The model under review builds one solid part; all positions refer to its coordinate system, in mm. Face numbers are marked on the shaded views. Give positions to 0.01 mm unless a question says otherwise; leave off trailing zeros. Loops run counter-clockwise (first coordinate to the right, second up) from the corner with the lowest first, then second, coordinate; pieces in that order, holes last. Notation, with made-up numbers: M 41,37.25 L 74,37.25 A20 cw 74,56.25 Z; hole C 60.5,-32 d5. An arc over 180 degrees is marked long. Put each result on its own line as item: value. Start each with the question number.
```python
from build123d import *

# Parameters (mm, degrees)
SKETCH1_R                               = 195
SKETCH1_R_2                             = 77.5
BOSS_EXTRUDE1_DEPTH                     = 5
SKETCH1_R_3                             = 67.5
SKETCH1_R_4                             = 25
BOSS_EXTRUDE1_2_DEPTH                   = 5
SKETCH1_4_R                             = 200
SKETCH1_4_R_2                           = 195
BOSS_EXTRUDE2_DEPTH                     = 147
SKETCH1_5_R                             = 77.5
SKETCH1_5_R_2                           = 67.5
BOSS_EXTRUDE3_DEPTH                     = 147
SKETCH1_6_R                             = 25
BOSS_EXTRUDE4_DEPTH                     = 25
BOSS_EXTRUDE5_DEPTH                     = 7
CBORE_FOR_M5_HEX_HEAD_BOLT1_D           = 5.8
CBORE_FOR_M5_HEX_HEAD_BOLT1_CBORE_D     = 12.238
CBORE_FOR_M5_HEX_HEAD_BOLT1_CBORE_DEPTH = 3.5
RIB1_REACH                              = 320.762
SKETCH4_WALLS_W                         = 10
SKETCH4_WALLS_H                         = 759.430387561
SKETCH4_WALLS_H_2                       = 759.674772851
SKETCH4_WALLS_W_2                       = 760.012833466
SKETCH4_WALLS_H_3                       = 10
SKETCH4_WALLS_W_3                       = 759.068922963
SKETCH5_R                               = 70
SKETCH5_R_2                             = 57.5
BOSS_EXTRUDE6_DEPTH                     = 29


with BuildPart() as part:
    # Sketch1 → Boss-Extrude1 (new body)
    with BuildSketch(Plane.XY):
        Circle(SKETCH1_R)
        Circle(SKETCH1_R_2, mode=Mode.SUBTRACT)
    extrude(amount=BOSS_EXTRUDE1_DEPTH)

    # Sketch1_4 → Boss-Extrude2 (add)
    with BuildSketch(Plane.XY):
        Circle(SKETCH1_4_R)
        Circle(SKETCH1_4_R_2, mode=Mode.SUBTRACT)
    extrude(amount=BOSS_EXTRUDE2_DEPTH)



with BuildPart() as body_2:
    # Sketch1 → Boss-Extrude1 2 (new body)
    with BuildSketch(Plane.XY):
        Circle(SKETCH1_R_3)
        Circle(SKETCH1_R_4, mode=Mode.SUBTRACT)
    extrude(amount=BOSS_EXTRUDE1_2_DEPTH)


with BuildPart() as part_1:
    add(part.part)

    add(body_2.part)  # Boss-Extrude3 merges body 2
    # Sketch1_5 → Boss-Extrude3 (add)
    with BuildSketch(Plane.XY):
        Circle(SKETCH1_5_R)
        Circle(SKETCH1_5_R_2, mode=Mode.SUBTRACT)
    extrude(amount=BOSS_EXTRUDE3_DEPTH)

    # Sketch1_6 → Boss-Extrude4 (add)
    with BuildSketch(Plane.XY):
        Circle(SKETCH1_6_R)
        with BuildLine():
            Line((-1.5, 11), (1.5, 11))
            ThreePointArc((1.5, 11), (2.207106781, 10.707106781), (2.5, 10))
            Line((2.5, 10), (2.5, 7.599342077))
            ThreePointArc((2.5, 7.599342077), (6.480740698, 4.69041576), (8, 0))
            ThreePointArc((8, 0), (-4.69041576, -6.480740698), (-2.5, 7.599342077))
            Line((-2.5, 7.599342077), (-2.5, 10))
            ThreePointArc((-2.5, 10), (-2.207106781, 10.707106781), (-1.5, 11))
        make_face(mode=Mode.SUBTRACT)
    extrude(amount=BOSS_EXTRUDE4_DEPTH)

    # Sketch1_7 → Boss-Extrude5 (add)
    with BuildSketch(Plane.XY):
        with BuildLine():
            ThreePointArc((8, 0), (6.480740698, 4.69041576), (2.5, 7.599342077))
            Line((2.5, 7.599342077), (2.5, 5))
            Line((2.5, 5), (-2.5, 5))
            Line((-2.5, 5), (-2.5, 7.599342077))
            ThreePointArc((-2.5, 7.599342077), (-4.69041576, -6.480740698), (8, 0))
        make_face()
        with BuildLine():
            Line((2.5, 5), (2.5, 7.599342077))
            ThreePointArc((2.5, 7.599342077), (0, 8), (-2.5, 7.599342077))
            Line((-2.5, 7.599342077), (-2.5, 5))
            Line((-2.5, 5), (2.5, 5))
        make_face()
        with BuildLine():
            ThreePointArc((2.5, 10), (2.207106781, 10.707106781), (1.5, 11))
            Line((1.5, 11), (-1.5, 11))
            ThreePointArc((-1.5, 11), (-2.207106781, 10.707106781), (-2.5, 10))
            Line((-2.5, 10), (-2.5, 7.599342077))
            ThreePointArc((-2.5, 7.599342077), (0, 8), (2.5, 7.599342077))
            Line((2.5, 7.599342077), (2.5, 10))
        make_face()
    extrude(amount=BOSS_EXTRUDE5_DEPTH)

    # CBORE for M5 Hex Head Bolt1 (through all)
    with Locations(Plane(origin=(0, 0, 0), x_dir=(-1, 0, 0), z_dir=(0, 0, -1))):
        with Locations((0, 0)):
            CounterBoreHole(CBORE_FOR_M5_HEX_HEAD_BOLT1_D / 2, CBORE_FOR_M5_HEX_HEAD_BOLT1_CBORE_D / 2, CBORE_FOR_M5_HEX_HEAD_BOLT1_CBORE_DEPTH)

    # Sketch4 walls → Rib1 (add, up to next)
    with BuildSketch(Plane.XY.offset(147), mode=Mode.PRIVATE) as rib1_sk1:
        with Locations((0, 137.453527328)):
            Rectangle(SKETCH4_WALLS_W, SKETCH4_WALLS_H)
    rib1_tool1 = extrude(rib1_sk1.sketch, amount=-RIB1_REACH, mode=Mode.PRIVATE) - part_1.part
    # Sketch4 walls → Rib1 (add, up to next)
    with BuildSketch(Plane.XY.offset(147), mode=Mode.PRIVATE) as rib1_sk2:
        with Locations((0, -137.575719973)):
            Rectangle(SKETCH4_WALLS_W, SKETCH4_WALLS_H_2)
    rib1_tool2 = extrude(rib1_sk2.sketch, amount=-RIB1_REACH, mode=Mode.PRIVATE) - part_1.part
    # Sketch4 walls → Rib1 (add, up to next)
    with BuildSketch(Plane.XY.offset(147), mode=Mode.PRIVATE) as rib1_sk3:
        with Locations((137.74475028, 0)):
            Rectangle(SKETCH4_WALLS_W_2, SKETCH4_WALLS_H_3)
    rib1_tool3 = extrude(rib1_sk3.sketch, amount=-RIB1_REACH, mode=Mode.PRIVATE) - part_1.part
    # Sketch4 walls → Rib1 (add, up to next)
    with BuildSketch(Plane.XY.offset(147), mode=Mode.PRIVATE) as rib1_sk4:
        with Locations((-137.272795029, 0)):
            Rectangle(SKETCH4_WALLS_W_3, SKETCH4_WALLS_H_3)
    rib1_tool4 = extrude(rib1_sk4.sketch, amount=-RIB1_REACH, mode=Mode.PRIVATE) - part_1.part
    add(rib1_tool1.solids().sort_by_distance((0, 137.453527328, 147))[0])
    add(rib1_tool2.solids().sort_by_distance((0, -137.575719973, 147))[0])
    add(rib1_tool3.solids().sort_by_distance((137.74475028, 0, 147))[0])
    add(rib1_tool4.solids().sort_by_distance((-137.272795028, 0, 147))[0])

    # Sketch5 → Boss-Extrude6 (add)
    with BuildSketch(Plane.XY.offset(5)):
        Circle(SKETCH5_R)
        with Locations(Location((0, 0, 0), (0, 0, 180))):
            Circle(SKETCH5_R_2, mode=Mode.SUBTRACT)
    extrude(amount=BOSS_EXTRUDE6_DEPTH)


solid = part_1.part
```
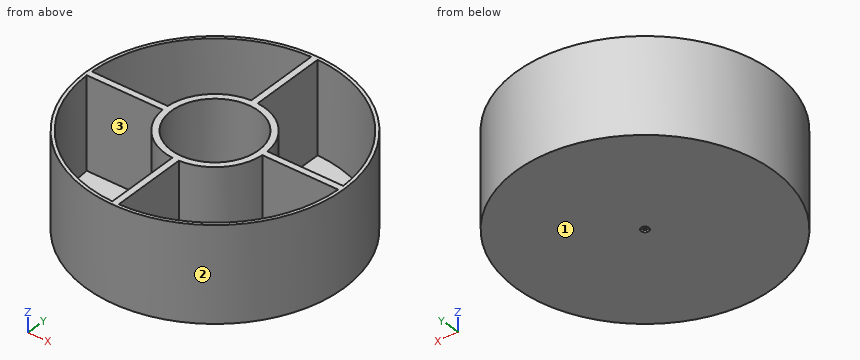
Item 1: To check wall thickness, follow L1, parallel to Y at x = 0, z = 20.5; L2, parallel to X at y = 61, z = 120; L3, parallel to Y at x = 48.5, z = 79.5. State the ranges of each line that lie inside material, in increasing order. Write a range as [from, to].
Item 2: Consider section C-C, the plane x = -33. Write out the cut boundary in (y, z), plus the area to 3 significant figures.
Item 3: Clearance check with flat-ended pins moving along their axes: pin 1 Ø1 at (y, z) = (-65.5, 81) entering from +X; pin 2 Ø5 at (x, z) = (39, 82.5) entering from -Y; pin 3 Ø19.5 at (x, y) = (0, 0) entering from -Z; pin 4 Ø6 at (x, y) = (-147, -121.5) entering from +Z. State where each tip first meets the part, or that it passes through.
Item 4: Draft analysis for pull direction X (two halves, no side actions). For the marked faces 1, 2 and 3, state which applies: +X half, -X half, draft (parallel to the pull), parting line (faces both ways), or undercut.
Item 5: Consider section D-D, the plane x = -95. Write out the cut boundary in (y, z).
Item 6: Consider section A-A, the plane z = 83. Write out the cut boundary in (x, y).
Item 7: Consider section B-B, the plane y = -43. Write out the cut boundary in (x, z).
Report:
1. L1: [-200, -57.5], [-25, -8], [11, 25], [57.5, 200]
1. L2: [-190.47, -185.21], [-47.8, -28.9], [28.9, 47.8], [185.21, 190.47]
1. L3: [-194.03, -188.87], [-60.45, -46.95], [46.95, 60.45], [188.87, 194.03]
2. outline: M -197.26,0 L 197.26,0 L 197.26,147 L 192.19,147 L 192.19,5 L 70.12,5 L 70.12,147 L 58.88,147 L 58.88,34 L 47.09,34 L 47.09,5 L -47.09,5 L -47.09,34 L -58.88,34 L -58.88,147 L -70.12,147 L -70.12,5 L -192.19,5 L -192.19,147 L -197.26,147 Z
2. area: 7,290 mm²
3. pin 1: x = 189.14
3. pin 2: y = -196.64
3. pin 3: z = 0
3. pin 4: z = 5
4. face 1: draft
4. face 2: parting line
4. face 3: undercut
5. outline: M -176,0 L 176,0 L 176,147 L 170.29,147 L 170.29,5 L 5,5 L 5,147 L -5,147 L -5,5 L -170.29,5 L -170.29,147 L -176,147 Z
6. outline: C 0,0 d400; hole M -194.94,-5 A195 ccw -5,-194.94 L -5,-77.34 A77.5 cw -77.34,-5 Z; hole M -194.94,5 L -77.34,5 A77.5 cw -5,77.34 L -5,194.94 A195 ccw Z; hole C 0,0 d135; hole M 5,-194.94 A195 ccw 194.94,-5 L 77.34,-5 A77.5 cw 5,-77.34 Z; hole M 5,77.34 A77.5 cw 77.34,5 L 194.94,5 A195 ccw 5,194.94 Z
7. outline: M -195.32,0 L 195.32,0 L 195.32,147 L 190.2,147 L 190.2,5 L 64.48,5 L 64.48,147 L 52.03,147 L 52.03,34 L 38.17,34 L 38.17,5 L -38.17,5 L -38.17,34 L -52.03,34 L -52.03,147 L -64.48,147 L -64.48,5 L -190.2,5 L -190.2,147 L -195.32,147 Z
